Autodesk Inventor part; units mm, degrees
ref_plane "Work Plane2" through (0, 8.5, 0) normal (0, -1, 0) x (1, 0, 0)
ref_plane "YZ Plane" through (0, 0, 0) normal (1, 0, 0) x (0, 1, 0)
ref_plane "XZ Plane" through (0, 0, 0) normal (0, 1, 0) x (-1, 0, 0)
sketch "Sketch1" plane through (0, 0, 0) normal (0, 0, 1) x (1, 0, 0)
  line L0 (0, 0) -> (0, 5)
  line L1 (0, 5) -> (24.5, 19.1451)
  line L2 (24.5, 19.1451) -> (44.5, 19.1451)
  line L3 (44.5, 19.1451) -> (69, 5)
  line L4 (69, 5) -> (69, 0)
  line L5 (69, 0) -> (44.5, 0)
  line L6 (44.5, 0) -> (44.5, -7)
  line L7 (44.5, -7) -> (24.5, -7)
  line L8 (24.5, -7) -> (24.5, 0)
  line L9 (24.5, 0) -> (0, 0)
  dimension "d0" = 20
  dimension "d1" = 7
  dimension "d2" = 5
  dimension "d3" = 24.5
  dimension "d4" = 120
  dimension "d5" = 120
  dimension "d6" = 20
extrude "Extrusion1" add sketch "Sketch1" along normal blind 20
sketch "Sketch2" plane through (24.5, -7, 0) normal (0, -1, 0) x (1, 0, 0)
  line L0 (0, 0) -> (20, 0)
  line L1 (20, 0) -> (20, 20)
  line L2 (0, 20) -> (20, 20)
  line L3 (0, 0) -> (0, 20)
  line L4 (0, 15) -> (2.5, 12.5)
  line L5 (2.5, 12.5) -> (2.5, 7.5)
  line L6 (2.5, 7.5) -> (0, 5)
  point P0 (-24.5, 0)
  point P1 (0, 10)
  point P2 (2.5, 10)
  dimension "d9" = 135
  dimension "d10" = 135
  dimension "d11" = 10
  dimension "d12" = 2.5
extrude "Extrusion2" cut sketch "Sketch2" against normal up to surface (7 mm away) contours L3 L4 L5 L6
ref_plane "Work Plane1" through (34.5, -7, 20) normal (-1, 0, 0) x (0, 0, 1)
sketch "Sketch3" plane through (0, 0, 0) normal (0, -1, 0) x (1, 0, 0)
  line L0 (24.5, 15) -> (24.5, 20)
  line L1 (0, 0) -> (0, 20)
  circle A0 centre (9.15, 10) radius 4
  circle A1 centre (9.15, 10) radius 1.6
  point P0 (0, 10)
  dimension "d15" = 15.35
  dimension "d16" = 3.2
  dimension "d17" = 8
extrude "Extrusion3" cut sketch "Sketch3" against normal through all contours A1
ref_plane "Work Plane2" through (0, 8.5, 0) normal (0, -1, 0) x (1, 0, 0)
extrude "Extrusion4" cut sketch "Sketch3" against normal blind 10 from surface at -8.5
sketch "Sketch4" plane through (24.5, 19.1451, 0) normal (0, 1, 0) x (1, 0, 0)
  line L0 (20, 0) -> (0, 0)
  line L1 (0, 0) -> (0, -20)
  line L2 (20, -20) -> (0, -20)
  line L3 (20, 0) -> (20, -20)
  point P0 (-24.5, 0)
  point P1 (10, -10)
  point P2 (20, -10)
  point P3 (10, -20)
hole "Hole1" at (34.5, 19.1451, 10) direction (0, -1, 0) diameter 6.2 end through all counterbore diameter 11 counterbore depth 19
mirror "Mirror1" about plane through (34.5, -7, 20) normal (-1, 0, 0) of "Extrusion2", "Extrusion3", "Extrusion4"
chamfer "Chamfer1" distance 6 angle 45 4 edges at (0, 2.5, 0) (0, 2.5, 20) (69, 2.5, 20) (69, 2.5, 0)
fillet "Fillet1" radius 2 14 edges at (3, 0, 3) (24.5, -7, 2.5) (24.5, -7, 17.5) (3, 0, 17) (3, 6.7321, 17) (3, 6.7321, 3) (24.5, 19.1451, 10) (44.5, -7, 17.5) (44.5, -7, 2.5) (66, 6.7321, 17) (66, 0, 17) (66, 6.7321, 3) (66, 0, 3) (44.5, 19.1451, 10)
chamfer "Chamfer2" distance 4 angle 45 4 edges at (58.4993, 11.0626, 13.7651) (58.4993, 11.0626, 6.2349) (10.5007, 11.0626, 6.2349) (10.5007, 11.0626, 13.7651)
properties part number "Belt tensioner mount"
The listing builds one solid part. Answer for the finished solid, in the listing's coordinates (mm). A direction names the side the tool comes from. Give positions to 0.01 mm unless a question says otherwise; leave off trailing zeros. Loops run counter-clockwise (first coordinate to the right, second up) from the corner with the lowest first, then second, coordinate; pieces in that order, holes last.
Item 1: A cutting plane is placed at C-C (y = 1). Give the vertices of the cut face in (x, z), then the cut area to 3 significant figures.
Derived:
outline: (0, 6.38) - (6.38, 0) - (62.62, 0) - (69, 6.38) - (69, 13.62) - (62.62, 20) - (6.38, 20) - (0, 13.62) - close; hole circle Ø3.2 at (9.15, 10); hole circle Ø11 at (34.5, 10); hole circle Ø3.2 at (59.85, 10)
area: 1,190 mm2
Item 2: Each of these flat-tipped pins is pushed along its axis until it touches: pin 1 Ø5 at (x, z) = (59.85, 10) entering from +Y; pin 2 Ø5 at (x, z) = (9.15, 10) entering from -Y; pin 3 Ø4 at (x, z) = (56, 9.5) entering from +Y. Where does it stop, or does it pass through?
Derived:
pin 1: stops at y = 8.5
pin 2: stops at y = 0
pin 3: stops at y = 11.83
Item 3: A cutting plane is placed at B-B (z = 10). Give the number of separate pieces and of enclosed holes in the cut face, then the cut area to 3 significant figures.
Derived:
separate pieces: 4
enclosed holes: 0
area: 729 mm2
Item 4: Find the intervals of material crossed by line 1 along Z through (x, y) = (9.15, 4.5); line 2 along Z through (x, y) = (34.5, 8.25); line 3 along X through (y, z) = (8, 9.75), in increasing order.
Derived:
line 1: z = 0 to 8.4, 11.6 to 20
line 2: z = 0 to 4.5, 15.5 to 20
line 3: x = 5.2 to 7.57, 10.73 to 29.01, 39.99 to 58.27, 61.43 to 63.8
Item 5: A tool of negligible diameter and unlimited length cuts with its end or side. For faces 5 (the flat face through (9, 8.5, 12)), 6 (the cylindrical face through (65.64, 0.57, 3.49)), 7 (the flat face through (25.7, -3.5, 13.8)), 8 (the flat face through (24.5, -3, 2)), 9 (the flat face through (43.3, -3.5, 6.2)), from which of +Z, -Z, +X, -X, +Y, -Y can it reach the whole face along a straight path? Write none if from no direction.
Derived:
face 5: -X, +Y
face 6: -Z, +X, -Y
face 7: -X, -Y
face 8: +Z, -Z, -X, -Y
face 9: +X, -Y
Item 6: A cutting plane is placed at D-D (x = 48). Give the vertices of the cut face in (y, z), then the cut area to 3 significant figures.
Derived:
outline: (0, 0) - (17.12, 0) - (17.12, 20) - (0, 20) - close
area: 342 mm2
Item 7: Determine the mould class of faces 1 (the cylindrical face through (3.49, 0.57, 3.36)), 2 (the cylindrical face through (8.8, 4.19, 8.44)), 3 (the cylindrical face through (3.47, 0.6, 16.66)), 4 (the flat face through (17.191, 14.925, 9.86)) for opening direction Z: +Z half, -Z half, draft (parallel to the pull), parting line (faces both ways), or undercut.
Derived:
face 1: -Z half
face 2: undercut
face 3: +Z half
face 4: draft
Item 8: A cutting plane is placed at A-A (x = 34.5). Give the vertices of the cut face in (y, z), then the cut area to 3 significant figures.
Derived:
outline: (-7, 0) - (19.15, 0) - (19.15, 4.5) - (0.15, 4.5) - (0.15, 6.9) - (-7, 6.9) - close; (-7, 13.1) - (0.15, 13.1) - (0.15, 15.5) - (19.15, 15.5) - (19.15, 20) - (-7, 20) - close
area: 270 mm2
